from build123d import *

# Parameters (mm, degrees)
SKETCH_R  = 3
PAD_DEPTH = 4


with BuildPart() as part:
    # Sketch → Pad (new body)
    with BuildSketch(Plane.XY):
        with BuildLine():
            Line((-78, 119.313708), (-78, -119.313708))
            ThreePointArc((-78, -119.313708), (-76.765367, -121.161468), (-74.585786, -120.727922))
            Line((-74.585786, -120.727922), (-58.585786, -104.727922))
            ThreePointArc((-58.585786, -104.727922), (-58.152241, -104.079075), (-58, -103.313708))
            Line((-58, -50), (-58, -103.313708))
            ThreePointArc((-57.414214, -48.585786), (-57.847759, -49.234633), (-58, -50))
            Line((-57.414214, -48.585786), (-19.414214, -10.585786))
            ThreePointArc((-18, -10), (-18.765367, -10.152241), (-19.414214, -10.585786))
            Line((-18, -10), (18, -10))
            ThreePointArc((19.414214, -10.585786), (18.765367, -10.152241), (18, -10))
            Line((19.414214, -10.585786), (57.414214, -48.585786))
            ThreePointArc((58, -50), (57.847759, -49.234633), (57.414214, -48.585786))
            Line((58, -50), (58, -103.313708))
            ThreePointArc((58, -103.313708), (58.152241, -104.079075), (58.585786, -104.727922))
            Line((58.585786, -104.727922), (74.585786, -120.727922))
            ThreePointArc((74.585786, -120.727922), (76.765367, -121.161468), (78, -119.313708))
            Line((78, -119.313708), (78, 119.313708))
            ThreePointArc((78, 119.313708), (76.765367, 121.161468), (74.585786, 120.727922))
            Line((58.585786, 104.727922), (74.585786, 120.727922))
            ThreePointArc((58.585786, 104.727922), (58.152241, 104.079075), (58, 103.313708))
            Line((58, 50), (58, 103.313708))
            ThreePointArc((57.414214, 48.585786), (57.847759, 49.234633), (58, 50))
            Line((19.414214, 10.585786), (57.414214, 48.585786))
            ThreePointArc((18, 10), (18.765367, 10.152241), (19.414214, 10.585786))
            Line((18, 10), (-18, 10))
            ThreePointArc((-19.414214, 10.585786), (-18.765367, 10.152241), (-18, 10))
            Line((-19.414214, 10.585786), (-57.414214, 48.585786))
            ThreePointArc((-58, 50), (-57.847759, 49.234633), (-57.414214, 48.585786))
            Line((-58, 50), (-58, 103.313708))
            ThreePointArc((-58, 103.313708), (-58.152241, 104.079075), (-58.585786, 104.727922))
            Line((-74.585786, 120.727922), (-58.585786, 104.727922))
            ThreePointArc((-74.585786, 120.727922), (-76.765367, 121.161468), (-78, 119.313708))
        make_face()
        with Locations((-68, 0)):
            Circle(SKETCH_R, mode=Mode.SUBTRACT)
        with Locations((68, 0)):
            Circle(SKETCH_R, mode=Mode.SUBTRACT)
        with Locations((-68, -100)):
            Circle(SKETCH_R, mode=Mode.SUBTRACT)
        with Locations((68, -100)):
            Circle(SKETCH_R, mode=Mode.SUBTRACT)
        Circle(SKETCH_R, mode=Mode.SUBTRACT)
        with Locations((-68, 100)):
            Circle(SKETCH_R, mode=Mode.SUBTRACT)
        with Locations((68, 100)):
            Circle(SKETCH_R, mode=Mode.SUBTRACT)
    extrude(amount=PAD_DEPTH)


solid = part.part
Can you work these out from the model? Positions are in its coordinate system, mm. A direction names the side the tool comes from. Coordinates: 2 decimals unless noted, no trailing zeros. Write each loop counter-clockwise with the first axis right and the second up, starting at its lowest first coordinate (ties: lowest second). Pieces come first, ordered by that corner, then holes. Notation, with made-up numbers: (6.5, -15.5) -> (43.5, -15.5) arc R16 ccw to (43.5, -0.5) -> close; hole circle Ø4 at (64.25, -33.75). An arc over 180 degrees is marked (long way). Write each question's results on one line, items separated by ' | '. Start each with the question number.
Q1. Imagine slicing it at C-C (x = -68). Write out the boundary of the cut face in (y, z).
Q2. On a 3-axis mill with a long thin cutter (end or side, diameter ignored), from which of +Z, -Z, +X, -X, +Y, -Y can I reach the whole of each face in a straight line? I mean faces 4 (the face through (-38.68, -29.85, 1.97)), 5 (the face through (38.15, 29.32, 1.97)), 6 (the face through (-68.65, 97.07, 1.97)). Say none if no direction works.
Q3. Imagine slicing it at D-D (y = 28.5). Write out the boundary of the cut face in (x, z), then the cut area to 3 significant figures.
Q4. We'd pull the mould along Y, two halves only. Please class faces 1 (the face through (-68.65, -102.93, 1.97)), 2 (the face through (-6.1, 9.6, 0)), 3 (the face through (-38.15, 29.32, 1.97)): +Y half, -Y half, draft (parallel to the pull), parting line (faces both ways), or undercut.
Q5. Imagine slicing it at B-B (x = 0). Write out the boundary of the cut face in (y, z).
Q6. If I drill on probe 1 along X at (y, z) = (-71, 1.55); probe 2 along Y at (x, z) = (68, 2.9); probe 3 along Y at (x, z) = (-16, 1), over which ranges is the centre line in solid material (lowest first)?
Q7. Imagine slicing it at A-A (y = 0). Write out the boundary of the cut face in (x, z), then the cut area to 3 significant figures.
Taken from the geometry:
1) outline: (-114.14, 0) -> (-103, 0) -> (-103, 4) -> (-114.14, 4) -> close; (-97, 0) -> (-3, 0) -> (-3, 4) -> (-97, 4) -> close; (3, 0) -> (97, 0) -> (97, 4) -> (3, 4) -> close; (103, 0) -> (114.14, 0) -> (114.14, 4) -> (103, 4) -> close
2) face 4: +Z, -Z, -Y | face 5: +Z, -Z, +Y | face 6: +Z, -Z
3) outline: (-78, 0) -> (-37.33, 0) -> (-37.33, 4) -> (-78, 4) -> close; (37.33, 0) -> (78, 0) -> (78, 4) -> (37.33, 4) -> close | area: 325 mm^2
4) face 1: undercut | face 2: draft | face 3: +Y half
5) outline: (-10, 0) -> (-3, 0) -> (-3, 4) -> (-10, 4) -> close; (3, 0) -> (10, 0) -> (10, 4) -> (3, 4) -> close
6) probe 1: x = -78 to -58, 58 to 78 | probe 2: y = -114.14 to -103, -97 to -3, 3 to 97, 103 to 114.14 | probe 3: y = -10 to 10
7) outline: (-78, 0) -> (-71, 0) -> (-71, 4) -> (-78, 4) -> close; (-65, 0) -> (-3, 0) -> (-3, 4) -> (-65, 4) -> close; (3, 0) -> (65, 0) -> (65, 4) -> (3, 4) -> close; (71, 0) -> (78, 0) -> (78, 4) -> (71, 4) -> close | area: 552 mm^2
